Model file for the job. Use its own axes, mm. Face numbers are marked on the shaded views. A direction names the side the tool comes from. Coordinates: 2 decimals unless noted, no trailing zeros. Loops run counter-clockwise (first coordinate to the right, second up) from the corner with the lowest first, then second, coordinate; pieces in that order, holes last. Notation, with made-up numbers: M 51,73.5 L 100,73.5 A18 cw 100,98.5 Z; hole C 39.25,53 d8. An arc over 180 degrees is marked long. One line per question, with ' | ' between items. Start each with the question number.
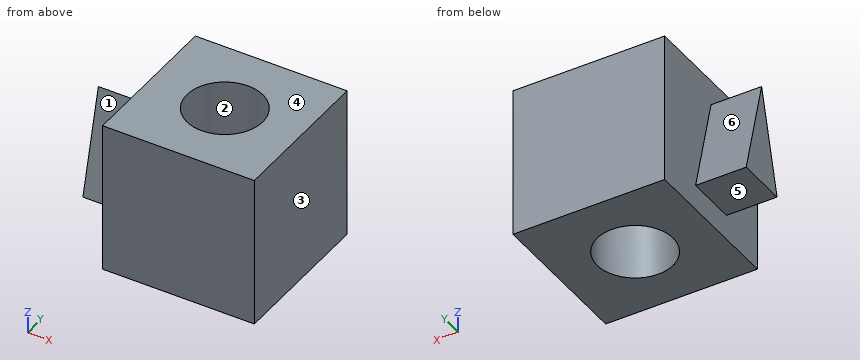
```python
from build123d import *

# Parameters (mm, degrees)
F0_W     = 152.4
F0_H     = 152.4
F1_DEPTH = 76.2
F2_R     = 38.1
F3_DEPTH = 152.401
F5_DEPTH = 50.8


with BuildPart() as f1:
    # F0 (on Top) → F1 (new body, symmetric)
    with BuildSketch(Plane.XY):
        Rectangle(F0_W, F0_H)
    extrude(amount=F1_DEPTH, both=True)

    # F2 (on face) → F3 (cut, through all)
    with BuildSketch(Plane.XY.offset(76.2)):
        Circle(F2_R)
    extrude(amount=-F3_DEPTH, mode=Mode.SUBTRACT)

    # F4 (on face) → F5 (join)
    with BuildSketch(Plane(origin=(-76.2, 0, 0), x_dir=(0, -1, 0), z_dir=(-1, 0, 0))):
        Polygon((0, 50.8), (-25.4, -50.8), (25.4, -50.8), align=None)
    extrude(amount=F5_DEPTH)


solid = f1.part
```
(1) Drill centre lines: line 1 (Y direction, x = 0, z = -19); line 2 (X direction, y = -55, z = 20.5); line 3 (X direction, y = -7.5, z = -64). Where is each one in solid material? Low to high. Write a range as [from, to].
(2) 3-axis set-ups, long thin cutter, end or side, ignore diameter. For the marked faces 4, 5 and 6: which of +Z, -Z, +X, -X, +Y, -Y reach the whole face in a straight line?
(3) Band-saw the part on D-D on z = 22. Write the cut outline in (x, y), then the cut area to 3 significant figures.
(4) Band-saw the part on C-C on z = 56.5. Write the cut outline in (x, y), then the cut area to 3 significant figures.
(5) Band-saw the part on B-B on y = -8.5. Write the cut outline in (x, z), then the cut area to 3 significant figures.
(6) Band-saw the part on A-A on x = 0. Write the cut outline in (y, z).
(7) Two-plate mould, pull along X, no slides. Class the marked faces 1, 2 and 3: pulls with the +X half, pulls with the -X half, needs draft (parallel to the pull), parting line crosses it, or undercut.
(8) Pin check, flat tips, straight feed: P1, Ø6, axis at y = 22.5, z = -6, coming from the -X side; P2, Ø2, axis at x = -94.5, y = 13, coming from the -Z side. Stop position of each tip, or through.
Computed values:
1) line 1: [-76.2, -38.1], [38.1, 76.2] | line 2: [-76.2, 76.2] | line 3: [-76.2, -37.35], [37.35, 76.2]
2) face 4: +Z, +X, -X, +Y, -Y | face 5: -Z, -X, +Y, -Y | face 6: +Z, -X, +Y
3) outline: M -127,-7.2 L -76.2,-7.2 L -76.2,-76.2 L 76.2,-76.2 L 76.2,76.2 L -76.2,76.2 L -76.2,7.2 L -127,7.2 Z; hole C 0,0 d76.2 | area: 19,400 mm^2
4) outline: M -76.2,-76.2 L 76.2,-76.2 L 76.2,76.2 L -76.2,76.2 Z; hole C 0,0 d76.2 | area: 18,700 mm^2
5) outline: M -127,-50.8 L -76.2,-50.8 L -76.2,-76.2 L -37.14,-76.2 L -37.14,76.2 L -76.2,76.2 L -76.2,16.8 L -127,16.8 Z; M 37.14,-76.2 L 76.2,-76.2 L 76.2,76.2 L 37.14,76.2 Z | area: 15,300 mm^2
6) outline: M -76.2,-76.2 L -38.1,-76.2 L -38.1,76.2 L -76.2,76.2 Z; M 38.1,-76.2 L 76.2,-76.2 L 76.2,76.2 L 38.1,76.2 Z
7) face 1: needs draft | face 2: undercut | face 3: pulls with the +X half
8) P1: x = -76.2 | P2: z = -50.8
